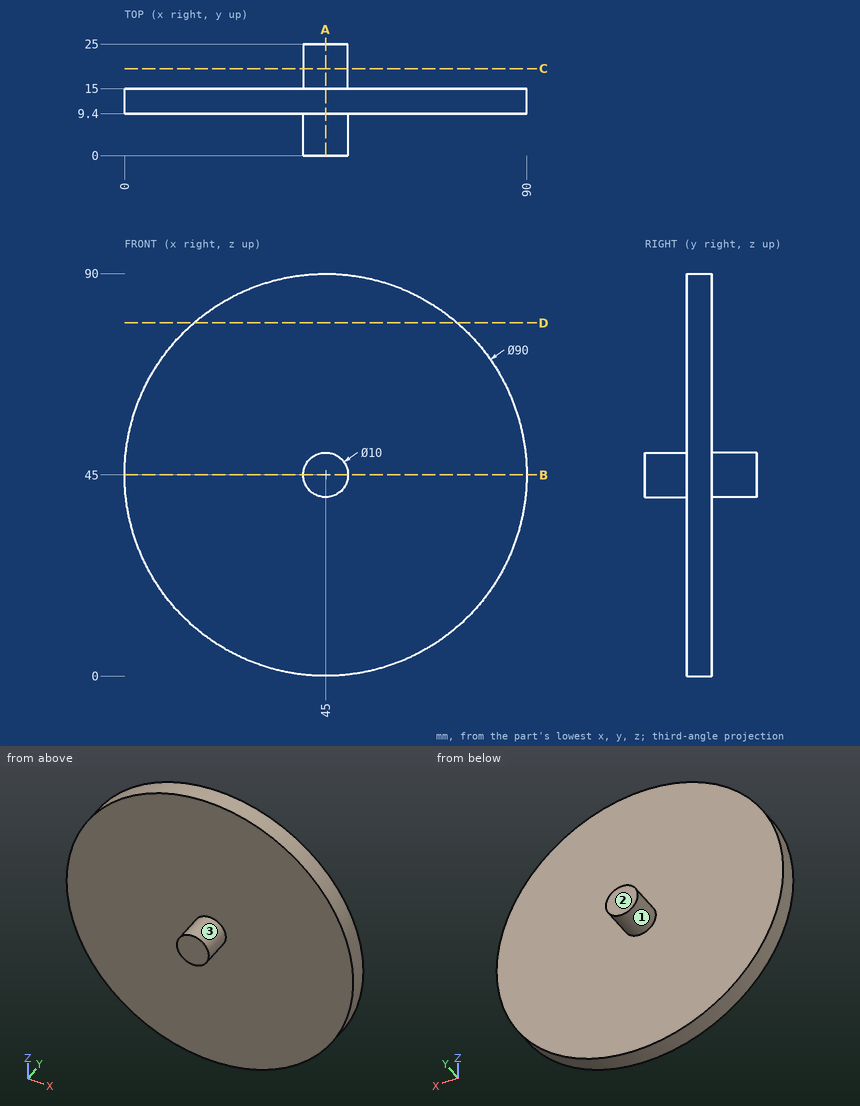
For this review, use the dimensioned drawing (mm, ordinates from the lowest corner) and the shaded views. A direction names the side the tool comes from. Coordinates: 2 decimals unless noted, no trailing zeros. Loops run counter-clockwise (first coordinate to the right, second up) from the corner with the lowest first, then second, coordinate; pieces in that order, holes last. Notation, with made-up numbers: (19.25, -28.5) - (37.25, -28.5) arc R15 cw to (37.25, -13.5) - close; hole circle Ø6 at (68, 61). An arc over 180 degrees is marked (long way). Use one line per item in the form item = value. Start each with the question number.
1) Take a section at D-D (z = 79). State the section outline as (x, y) points.
2) To check wall thickness, follow probe 1 along Y at (x, z) = (69, 23.5); probe 2 along X at (y, z) = (4.5, 45); probe 3 along X at (y, z) = (14.25, 57.5). State the ranges of each line that lie inside material, in increasing order. Write a range as from..to.
3) Take a section at C-C (y = 19.5). State the section outline as (x, z) points.
4) For the marked faces 1, 2 and 3, list the 3-axis set-ups (+Z, -Z, +X, -X, +Y, -Y) from which the entire face can be reached by the end or side of a thin tool; tool diameter is ignored.
5) For pin 1 (8 mm diameter, centred on y = 14, z = 40.5, fed in from +X); pin 2 (2 mm diameter, centred on x = 11, z = 72, fed in from -Y); pin 3 (12 mm diameter, centred on y = 16.5, z = 32, fed in from +X), all flat-tipped, find the tip position at first contact; note any pin that passes through.
6) Take a section at A-A (x = 45). State the section outline as (y, z) points.
7) Take a section at B-B (z = 45). State the section outline as (x, y) points.
From the geometry:
q1.outline = (15.52, 9.4) - (74.48, 9.4) - (74.48, 15) - (15.52, 15) - close
q2.probe_1 = 9.4..15
q2.probe_2 = 40..50
q2.probe_3 = 1.77..88.23
q3.outline = circle Ø10 at (45, 45)
q4.face_1 = +Y
q4.face_2 = +Z, -Z, +X, -X, +Y
q4.face_3 = -Y
q5.pin_1 = 90
q5.pin_2 = 9.4
q5.pin_3 = 89.42
q6.outline = (0, 40) - (9.4, 40) - (9.4, 0) - (15, 0) - (15, 40) - (25, 40) - (25, 50) - (15, 50) - (15, 90) - (9.4, 90) - (9.4, 50) - (0, 50) - close
q7.outline = (0, 9.4) - (40, 9.4) - (40, 0) - (50, 0) - (50, 9.4) - (90, 9.4) - (90, 15) - (50, 15) - (50, 25) - (40, 25) - (40, 15) - (0, 15) - close
